Source: CAD feature listing. Evaluate the final solid. Frame: model axes, mm. Give positions to 0.01 mm unless a question says otherwise; leave off trailing zeros. Put each result on its own line as item: value.
```python
from build123d import *

# Parameters (mm, degrees)
F0_W           = 171
F0_H           = 200
F1_DEPTH       = 18
F3_DEPTH       = 171.001
F5_D           = 3
F5_CSINK_D     = 8.2
F5_CSINK_ANGLE = 90
F6_D           = 3
F6_CSINK_D     = 8.2
F6_CSINK_ANGLE = 90


with BuildPart() as f1:
    # F0 (on Top) → F1 (new body)
    with BuildSketch(Plane.XY):
        Rectangle(F0_W, F0_H)
    extrude(amount=F1_DEPTH)

    # F2 (on face) → F3 (cut, through all)
    with BuildSketch(Plane.YZ.offset(85.5)):
        Polygon((100, 0), (100, 18), (96.826114, 0), align=None)
    extrude(amount=-F3_DEPTH, mode=Mode.SUBTRACT)

    # F5 (through all)
    with Locations(Plane.XY.offset(18)):
        with Locations((-76.5, 49.466), (76.5, 49.466)):
            CounterSinkHole(F5_D / 2, F5_CSINK_D / 2, counter_sink_angle=F5_CSINK_ANGLE)

    # F6 (through all)
    with Locations(Plane.XY.offset(18)):
        with Locations((-76.5, -40.534), (76.5, -40.534)):
            CounterSinkHole(F6_D / 2, F6_CSINK_D / 2, counter_sink_angle=F6_CSINK_ANGLE)


solid = f1.part
```
(1) Line query: probe 1 along Y at (x, z) = (76.5, 3); probe 2 along Y at (x, z) = (76.5, 10); probe 3 along Y at (x, z) = (29.5, 8.5). Output: solid intervals per line, ascending. Write a range as from..to.
Calculated:
probe 1: y = -100..-42.03, -39.03..47.97, 50.97..97.36
probe 2: y = -100..-42.03, -39.03..47.97, 50.97..98.59
probe 3: y = -100..98.32
(2) First-contact query: P1, Ø4, axis at x = 76.5, y = 49.466, coming from the +Z side; P2, Ø5, axis at x = 48, z = 9.5, coming from the +Y side. Flat tips, straight axial feed; report the tip coordinate or a pass-through.
Calculated:
P1: stops at z = 15.9
P2: stops at y = 98.94
(3) Draft query along Y for faces 1 (the conical face through (-78.002, -41.157, 15.526)), 2 (the flat face through (-1, -100, 9)), 3 (the flat face through (-1, 1, 18)). Return one class per face: released by +Y, released by -Y, zero draft, split by the parting line, or undercut.
Calculated:
face 1: undercut
face 2: released by -Y
face 3: zero draft
